Can you work these out from the drawing? Everything is in mm from the part's minimum corner. A direction names the side the tool comes from. Round coordinates to 2 decimals unless told otherwise and drop trailing zeros. Loops run counter-clockwise (first coordinate to the right, second up) from the corner with the lowest first, then second, coordinate; pieces in that order, holes last. Notation, with made-up numbers: M 51.25,62 L 73.25,62 A18 ccw 73.25,89 Z; hole C 16,85 d4. An arc over 180 degrees is marked long. Use a Markdown table: item, result.
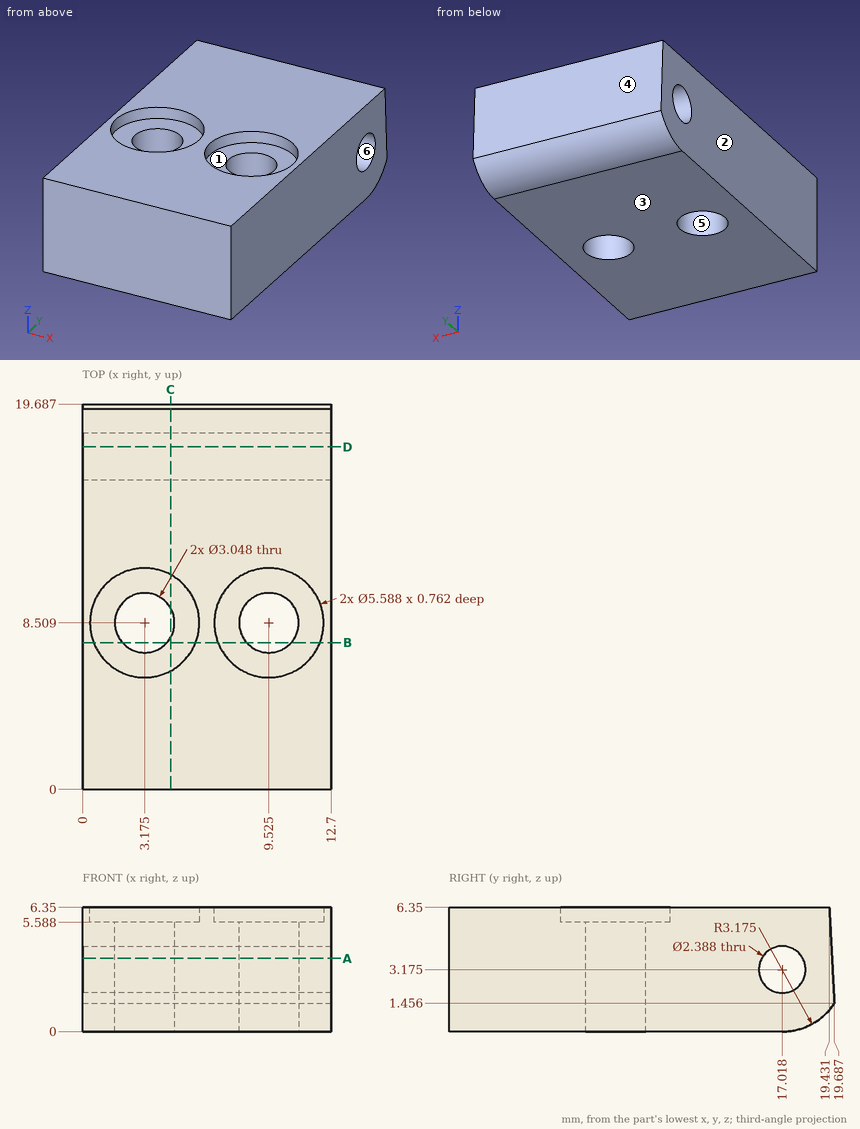
1. We'd pull the mould along Z, two halves only. Please class the marked faces 3, 4, 5 and 6: +Z half, -Z half, draft (parallel to the pull), parting line (faces both ways), or undercut.
Answer sheet:
| item | result |
|---|---|
| face 3 | -Z half |
| face 4 | +Z half |
| face 5 | draft |
| face 6 | undercut |
2. For pin 1 Ø4.5 at (x, y) = (3.175, 8.509) entering from +Z; pin 2 Ø2.5 at (x, y) = (9.525, 8.509) entering from +Z, each with a flat end and sliding along its axis, tell me the tip position at first contact or that it passes through.
Answer sheet:
| item | result |
|---|---|
| pin 1 | z = 5.59 |
| pin 2 | through |
3. I need wall thicknesses on probe 1 along Y at (x, z) = (3.5, 2.75) (1 decimal); probe 2 along Z at (x, y) = (7, 17); probe 3 along X at (y, z) = (8.25, 1.25). Which ranges of each line are inside material? Lowest first, please. Write a range as from..to.
Answer sheet:
| item | result |
|---|---|
| probe 1 | 0..7, 10..15.9, 18.1..19.6 |
| probe 2 | 0..1.98, 4.37..6.35 |
| probe 3 | 0..1.67, 4.68..8.02, 11.03..12.7 |
4. Imagine slicing it at D-D, the plane y = 17.5. Write out the boundary of the cut face in (x, z).
Answer sheet:
| item | result |
|---|---|
| outline | M 0,0.04 L 12.7,0.04 L 12.7,2.08 L 0,2.08 Z; M 0,4.27 L 12.7,4.27 L 12.7,6.35 L 0,6.35 Z |
5. Imagine slicing it at C-C, the plane x = 4.5. State how many separate pieces and enclosed holes the cut face has, then the cut area to 3 significant figures.
Answer sheet:
| item | result |
|---|---|
| separate pieces | 2 |
| enclosed holes | 1 |
| area | 107 mm2 |
6. Which directions (+Z, -Z, +X, -X, +Y, -Y) give clear straight access to the entire face, cutting with the end or side of a thin tool? Please do the marked faces 1 and 2.
Answer sheet:
| item | result |
|---|---|
| face 1 | +Z |
| face 2 | +Z, -Z, -X, +Y, -Y |
7. Imagine slicing it at B-B, the plane y = 7.5. Write out the boundary of the cut face in (x, z).
Answer sheet:
| item | result |
|---|---|
| outline | M 0,0 L 2.03,0 L 2.03,5.59 L 0.57,5.59 L 0.57,6.35 L 0,6.35 Z; M 4.32,0 L 8.38,0 L 8.38,5.59 L 6.92,5.59 L 6.92,6.35 L 5.78,6.35 L 5.78,5.59 L 4.32,5.59 Z; M 10.67,0 L 12.7,0 L 12.7,6.35 L 12.13,6.35 L 12.13,5.59 L 10.67,5.59 Z |
8. Imagine slicing it at A-A, the plane z = 3.75. Write out the boundary of the cut face in (x, y) (1 decimal), then the cut area to 3 significant figures.
Answer sheet:
| item | result |
|---|---|
| outline | M 0,0 L 12.7,0 L 12.7,16 L 0,16 Z; M 0,18.1 L 12.7,18.1 L 12.7,19.6 L 0,19.6 Z; hole C 3.2,8.5 d3; hole C 9.5,8.5 d3 |
| area | 207 mm2 |
